The figure shows three views and two pictorial views of one solid part (mm, origin at its lowest corner). Answer the questions. A direction names the side the tool comes from. Coordinates: 2 decimals unless noted, no trailing zeros. Loops run counter-clockwise (first coordinate to the right, second up) from the corner with the lowest first, then second, coordinate; pieces in that order, holes last. Notation, with made-up numbers: (26, 3) -> (39, 3) arc R12 ccw to (39, 7) -> close; hole circle Ø1 at (28.25, -1). An arc over 180 degrees is marked (long way). Answer in a Markdown table with one row per item.
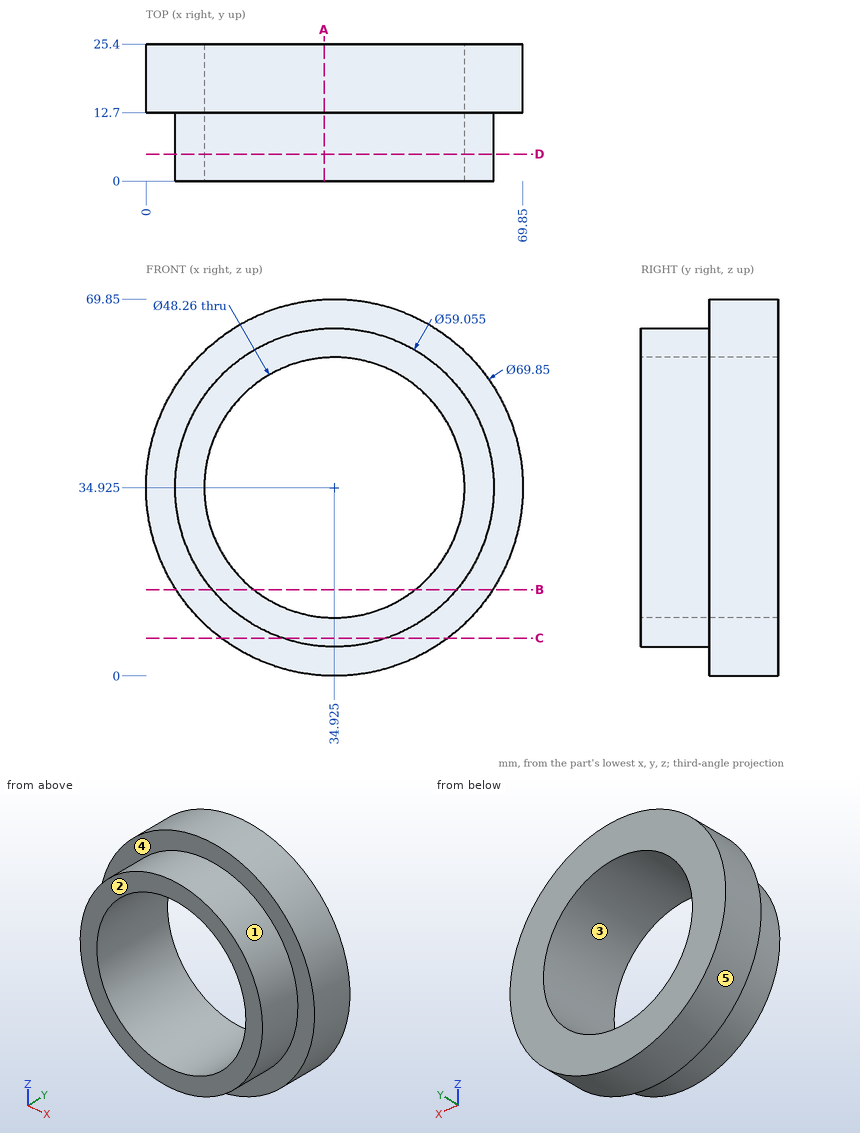
Item 1: A cutting plane is placed at A-A, the plane x = 33. Determine the outline of the cut face in (y, z), plus the area to 3 significant figures.
Findings below:
| item | result |
|---|---|
| outline | (0, 5.46) -> (12.7, 5.46) -> (12.7, 0.05) -> (25.4, 0.05) -> (25.4, 10.87) -> (0, 10.87) -> close; (0, 58.98) -> (25.4, 58.98) -> (25.4, 69.8) -> (12.7, 69.8) -> (12.7, 64.39) -> (0, 64.39) -> close |
| area | 412 mm2 |
Item 2: A cutting plane is placed at C-C, the plane z = 7. Determine the outline of the cut face in (x, y).
Findings below:
| item | result |
|---|---|
| outline | (13.95, 12.7) -> (25.33, 12.7) -> (25.33, 0) -> (44.52, 0) -> (44.52, 12.7) -> (55.9, 12.7) -> (55.9, 25.4) -> (13.95, 25.4) -> close |
Item 3: A tool of negligible diameter and unlimited length cuts with its end or side. For the marked faces 1 and 2, from which of +Z, -Z, +X, -X, +Y, -Y can it reach the whole face along a straight path? Write none if from no direction.
Findings below:
| item | result |
|---|---|
| face 1 | -Y |
| face 2 | +Z, -Z, +X, -X, -Y |
Item 4: A cutting plane is placed at B-B, the plane z = 16. Determine the outline of the cut face in (x, y).
Findings below:
| item | result |
|---|---|
| outline | (5.57, 12.7) -> (12.26, 12.7) -> (12.26, 0) -> (19.95, 0) -> (19.95, 25.4) -> (5.57, 25.4) -> close; (49.9, 0) -> (57.59, 0) -> (57.59, 12.7) -> (64.28, 12.7) -> (64.28, 25.4) -> (49.9, 25.4) -> close |
Item 5: Determine the mould class of the marked faces 3, 4 and 5 for opening direction X: +X half, -X half, draft (parallel to the pull), parting line (faces both ways), or undercut.
Findings below:
| item | result |
|---|---|
| face 3 | undercut |
| face 4 | draft |
| face 5 | parting line |
Item 6: Flat-ended cylindrical pins translate along their axes: pin 1 Ø5 at (x, y) = (27, 12.5) entering from -Z; pin 2 Ø10 at (y, z) = (22, 31.5) entering from -X; pin 3 Ø5 at (y, z) = (14, 37) entering from +X; pin 4 Ø12 at (x, z) = (41.5, 21.5) entering from -Y. Find the tip coordinate at first contact, or state that the pin passes through.
Findings below:
| item | result |
|---|---|
| pin 1 | stops at z = 0.43 |
| pin 2 | stops at x = 0 |
| pin 3 | stops at x = 69.85 |
| pin 4 | passes through |
Item 7: A cutting plane is placed at D-D, the plane y = 5. Determine the outline of the cut face in (x, z) (1 decimal).
Findings below:
| item | result |
|---|---|
| outline | circle Ø59.1 at (34.9, 34.9); hole circle Ø48.3 at (34.9, 34.9) |
Item 8: Find the intervals of material crossed by probe 1 along X at (y, z) = (19.75, 34); probe 2 along Y at (x, z) = (6.5, 51.5); probe 3 along X at (y, z) = (13.75, 15), in increasing order.
Findings below:
| item | result |
|---|---|
| probe 1 | x = 0.01 to 10.81, 59.04 to 69.84 |
| probe 2 | y = 12.7 to 25.4 |
| probe 3 | x = 6.24 to 21.31, 48.54 to 63.61 |
